Here's how the part is built. I have some questions about the finished solid (model axes, mm). A direction names the side the tool comes from. Give positions to 0.01 mm unless a question says otherwise; leave off trailing zeros. Loops run counter-clockwise (first coordinate to the right, second up) from the corner with the lowest first, then second, coordinate; pieces in that order, holes last. Notation, with made-up numbers: (70, 1.5) - (107, 1.5) arc R23 cw to (107, 9.5) - close; hole circle Ø11 at (-32.75, 34). An arc over 180 degrees is marked (long way). One line per item, written item: value. Start each with the question number.
```python
from build123d import *

# Parameters (mm, degrees)
BOSS_EXTRUDE1_DEPTH = 6.35
CAVITY1_START       = -6.35
CAVITY1_OUTLINE_R   = 12.7
CAVITY1_DEPTH       = 12.7


# Read off the part's stored shape, not the designer's step: Cavity1
with BuildPart() as part:
    # Sketch1 → Boss-Extrude1 (new, symmetric)
    with BuildSketch(Plane.XY):
        Polygon((785.7, 533.4), (785.7, 381), (732.36, 381), (732.36, 685.8), (785.7, 685.8), (1001.6, 685.8), (1087.96, 685.8), (1087.96, 381), (1014.3, 381), (1014.3, 533.4), (1001.6, 533.4), (1001.6, 381), (798.4, 381), (798.4, 533.4), align=None)
    extrude(amount=BOSS_EXTRUDE1_DEPTH, both=True)

    # Cavity1 outline → Cavity1 (cut)
    with BuildSketch(Plane.XY.offset(CAVITY1_START)):
        with Locations((900, 503.049546279)):
            Circle(CAVITY1_OUTLINE_R)
    extrude(amount=CAVITY1_DEPTH, mode=Mode.SUBTRACT)


solid = part.part
```
(1) For faces 1 (the face through (913, 536, 6.35)), 2 (the face through (1008, 533.4, 0)), which set-ups out of +Z, -Z, +X, -X, +Y, -Y let a thin tool reach every point of the face, with its end or its side?
(2) If we mould it in two halves opening along X, with no side actions, what happens to faces 3 (the face through (732.36, 531, 0)), 4 (the face through (913, 685.8, 0)), 5 (the face through (889.922, 495.322, -0.089))? For each: pulls with the +X half, pulls with the -X half, needs draft (parallel to the pull), parting line crosses it, or undercut.
(3) Please list where these lines run through material, in increasing order: probe 1 along X at (y, z) = (398, 0); probe 2 along Y at (x, z) = (900, -0.5); probe 3 along Y at (x, z) = (1006.5, 2.75). Write a range as from..to.
(4) If we section it at A-A on x = 900: List the corners of the cut face in (y, z) for me.
(5) Will this pin go through, and if not, where does the flat tip stop? pin 1 (6.5 mm diameter, centred on x = 794.5, z = -1.5, fed in from -Y).
(6) If we section it at B-B on z = 1.5: List the corners of the cut face in (x, y) for me, plus the area to 3 significant figures.
Found:
1. face 1: +Z, +X, -X, +Y, -Y
1. face 2: +Z, -Z, -Y
2. face 3: pulls with the -X half
2. face 4: needs draft
2. face 5: undercut
3. probe 1: 732.36..785.7, 798.4..1001.6, 1014.3..1087.96
3. probe 2: 381..490.35, 515.75..685.8
3. probe 3: 533.4..685.8
4. outline: (381, -6.35) - (490.35, -6.35) - (490.35, 6.35) - (381, 6.35) - close; (515.75, -6.35) - (685.8, -6.35) - (685.8, 6.35) - (515.75, 6.35) - close
5. pin 1: y = 533.4
6. outline: (732.36, 381) - (785.7, 381) - (785.7, 533.4) - (798.4, 533.4) - (798.4, 381) - (1001.6, 381) - (1001.6, 533.4) - (1014.3, 533.4) - (1014.3, 381) - (1087.96, 381) - (1087.96, 685.8) - (732.36, 685.8) - close; hole circle Ø25.4 at (900, 503.05)
6. area: 104,000 mm^2
